from build123d import *

# Parameters (mm, degrees)
SCHNITT_LINEAR_AUSTRAGEN1_DEPTH = 1.8
FASE1_SIZE                      = 0.2
VERRUNDUNG1_R                   = 0.2
VERRUNDUNG2_R                   = 0.1


with BuildPart() as part:
    # Skizze1 → Rotation1 (revolve)
    with BuildSketch(Plane(origin=(0, 0, 0), x_dir=(0, 0, -1), z_dir=(1, 0, 0))):
        Polygon((-3, 0), (-3, 2.75), (0, 2.75), (0, 1.465), (14, 1.465), (14, 0), align=None)
    revolve(axis=Axis((0, 0, 21.919879518), (0, 0, -1)))

    # Skizze2 → Schnitt-Linear austragen1 (cut)
    with BuildSketch(Plane.XY.offset(3)):
        Polygon((1.25, -0.721687836), (1.25, 0.721687836), (0, 1.443375673), (-1.25, 0.721687836), (-1.25, -0.721687836), (0, -1.443375673), align=None)
    extrude(amount=-SCHNITT_LINEAR_AUSTRAGEN1_DEPTH, mode=Mode.SUBTRACT)

    # Fase1
    fase1_edges = [part.edges().sort_by_distance(p)[0] for p in [
        (0, -1.465, -14),
        (0, -2.75, 0),
        (0, -2.75, 3),
    ]]
    chamfer(fase1_edges, length=FASE1_SIZE)

    # Verrundung1
    verrundung1_edges = [part.edges().sort_by_distance(p)[0] for p in [
        (0.625, -1.082531755, 1.2),
        (1.25, -0.721687836, 2.1),
        (-0.625, -1.082531755, 1.2),
        (0, -1.443375673, 2.1),
        (-1.25, 0, 1.2),
        (-1.25, -0.721687836, 2.1),
        (-0.625, 1.082531755, 1.2),
        (-1.25, 0.721687836, 2.1),
        (0.625, 1.082531755, 1.2),
        (0, 1.443375673, 2.1),
        (1.25, 0, 1.2),
        (1.25, 0.721687836, 2.1),
        (0, -1.465, 0),
    ]]
    fillet(verrundung1_edges, radius=VERRUNDUNG1_R)

    # Verrundung2
    verrundung2_edges = [part.edges().sort_by_distance(p)[0] for p in [
        (-0.625, -1.082531755, 3),
        (-1.25, 0, 3),
        (-0.625, 1.082531755, 3),
        (0.625, 1.082531755, 3),
        (1.25, 0, 3),
        (0.625, -1.082531755, 3),
        (-1.223205081, -0.706217783, 3),
        (0, -1.412435565, 3),
        (1.223205081, -0.706217783, 3),
        (1.223205081, 0.706217783, 3),
        (0, 1.412435565, 3),
        (-1.223205081, 0.706217783, 3),
    ]]
    fillet(verrundung2_edges, radius=VERRUNDUNG2_R)


solid = part.part
Model file for the job. Use its own axes, mm. A direction names the side the tool comes from. Give positions to 0.01 mm unless a question says otherwise; leave off trailing zeros. Write each loop counter-clockwise with the first axis right and the second up, starting at its lowest first coordinate (ties: lowest second). Pieces come first, ordered by that corner, then holes. Notation, with made-up numbers: (-14, -34) -> (-2, -34) arc R22 ccw to (-2, 1) -> close; hole circle Ø8 at (50.5, -29.75). An arc over 180 degrees is marked (long way). Write item = value, one per line.
(1) Flat gauge pins, fed straight in: P1, Ø1.5, axis at x = -2, z = -11.5, coming from the -Y side; P2, Ø2, axis at x = 0.5, z = -12, coming from the +Y side (3 decimals). Where does each tip first touch, or does it go through?
Determined:
P1 = -0.76
P2 = 1.465
(2) Tool access for faces 4 (the face through (-1, 2, 0)), 5 (the face through (0, 0, -14)), 6 (the face through (-0.63, -1.08, 2.16)): list every direction of +Z, -Z, +X, -X, +Y, -Y with a clear straight run to the whole face (end or side of a thin tool).
Determined:
face_4 = -Z
face_5 = -Z, +X, -X, +Y, -Y
face_6 = +Z
(3) Slice it at A-A, the plane y = 0. Give the cut face in (x, z) (3 decimals), then the cut area to 3 significant figures.
Determined:
outline = (-2.75, 0.2) -> (-2.55, 0) -> (-1.665, 0) arc R0.2 cw to (-1.465, -0.2) -> (-1.465, -13.8) -> (-1.265, -14) -> (1.265, -14) -> (1.465, -13.8) -> (1.465, -0.2) arc R0.2 cw to (1.665, 0) -> (2.55, 0) -> (2.75, 0.2) -> (2.75, 2.8) -> (2.55, 3) -> (1.35, 3) arc R0.1 ccw to (1.25, 2.9) -> (1.25, 1.4) arc R0.2 cw to (1.05, 1.2) -> (-1.05, 1.2) arc R0.2 cw to (-1.25, 1.4) -> (-1.25, 2.9) arc R0.1 ccw to (-1.35, 3) -> (-2.55, 3) -> (-2.75, 2.8) -> close
area = 52.9 mm2
(4) Probe line 1 along Z through (x, y) = (2.3, -0.7); line 2 along Z through (x, y) = (-0.7, 0.25); line 3 along Y through (x, z) = (-0.4, -5.75). List the from-to ranges inside material, lowest first.
Determined:
line_1 = 0 to 3
line_2 = -14 to 1.2
line_3 = -1.41 to 1.41
(5) Slice it at C-C, the plane z = -12.25. Give the cut face in (x, y) (3 decimals).
Determined:
outline = circle Ø2.93 at (0, 0)
(6) Mould opens along Y. For faces 1 (the face through (-1.1, -1.1, 3)), 2 (the face through (0.63, 1.08, 2.16)), 3 (the face through (-2.685, -0.596, 1.482)) say: released by +Y, released by -Y, zero draft, split by the parting line, or undercut.
Determined:
face_1 = zero draft
face_2 = undercut
face_3 = split by the parting line
(7) Slice it at B-B, the plane z = 1.75. Give the cut face in (x, y).
Determined:
outline = circle Ø5.5 at (0, 0); hole (-1.25, -0.61) arc R0.2 ccw to (-1.15, -0.78) -> (-0.1, -1.39) arc R0.2 ccw to (0.1, -1.39) -> (1.15, -0.78) arc R0.2 ccw to (1.25, -0.61) -> (1.25, 0.61) arc R0.2 ccw to (1.15, 0.78) -> (0.1, 1.39) arc R0.2 ccw to (-0.1, 1.39) -> (-1.15, 0.78) arc R0.2 ccw to (-1.25, 0.61) -> close
